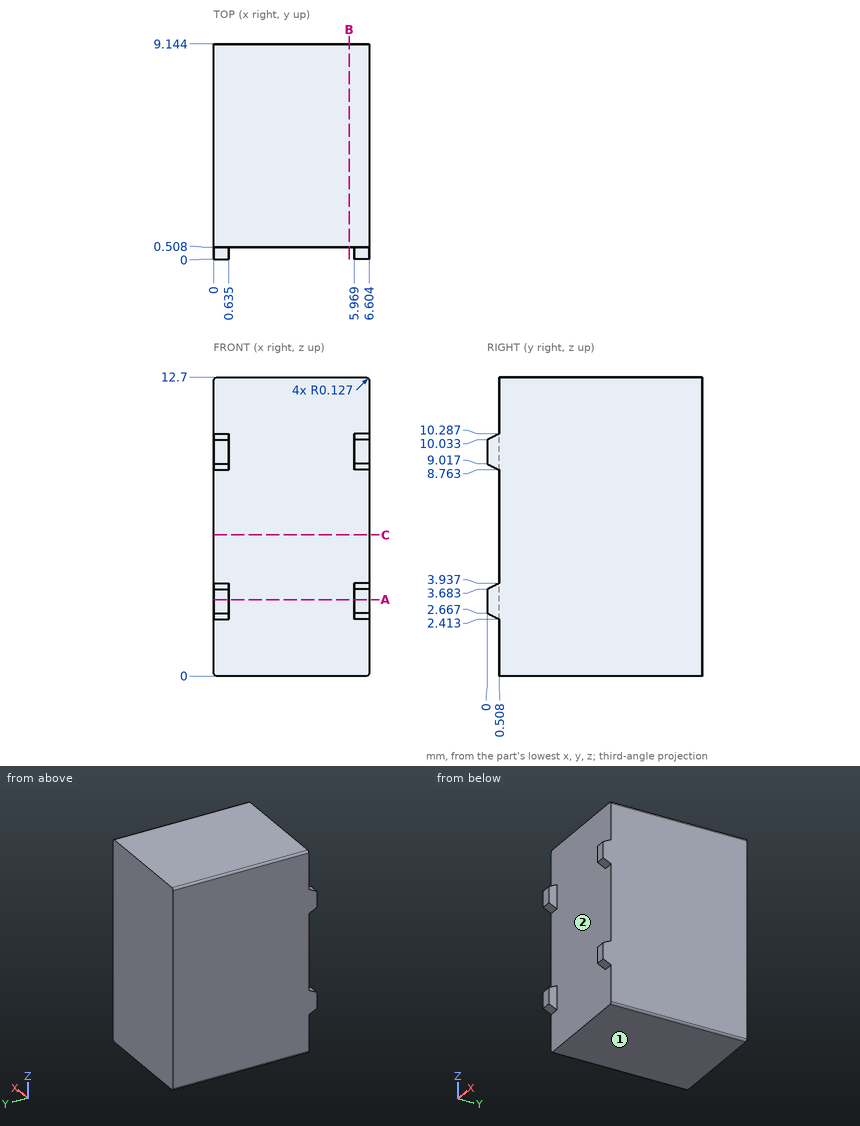
Here's the drawing with two shaded views (mm, measured from the low corner). I have some questions. A direction names the side the tool comes from. Give positions to 0.01 mm unless a question says otherwise; leave off trailing zeros. Write each loop counter-clockwise with the first axis right and the second up, starting at its lowest first coordinate (ties: lowest second). Pieces come first, ordered by that corner, then holes. Notation, with made-up numbers: (-21, -8) -> (1, -8) arc R14 ccw to (1, 8) -> close; hole circle Ø6 at (54, 84.25). An arc over 180 degrees is marked (long way). One line per item, written item: value.
Q1. Imagine slicing it at A-A on z = 3.25. Please give me the cut outline in (x, y) (3 decimals), and give its area (3 significant figures).
Results found:
outline: (0, 0) -> (0.635, 0) -> (0.635, 0.508) -> (5.969, 0.508) -> (5.969, 0) -> (6.604, 0) -> (6.604, 9.144) -> (0, 9.144) -> close
area: 57.7 mm^2
Q2. Which directions (+Z, -Z, +X, -X, +Y, -Y) give clear straight access to the entire face, cutting with the end or side of a thin tool? Please do the marked faces 1 and 2.
Results found:
face 1: -Z, +X, -X, +Y, -Y
face 2: -Y
Q3. Imagine slicing it at C-C on z = 6. Please give me the cut outline in (x, y).
Results found:
outline: (0, 0.51) -> (6.6, 0.51) -> (6.6, 9.14) -> (0, 9.14) -> close
Q4. For P1, Ø1, axis at x = 6, z = 5, coming from the -Y side; P2, Ø2, axis at x = 5.5, y = 8, coming from the -Z side, each with a flat end and sliding along its axis, tell me the tip position at first contact or that it passes through.
Results found:
P1: stops at y = 0.51
P2: stops at z = 0
Q5. Imagine slicing it at B-B on x = 5.75. Please give me the cut outline in (y, z).
Results found:
outline: (0.51, 0) -> (9.14, 0) -> (9.14, 12.7) -> (0.51, 12.7) -> close
Q6. Please list where this line runs through material, in increasing order: line 1 (Y direction, x = 3.5, z = 2.5). Write a range as [from, to].
Results found:
line 1: y = [0.51, 9.14]
